Input: part model. Units: mm. Frame: model coordinates. A direction names the side the tool comes from. Round coordinates to 2 decimals unless told otherwise and drop trailing zeros. Loops run counter-clockwise (first coordinate to the right, second up) from the corner with the lowest first, then second, coordinate; pieces in that order, holes last.
1) Access query for faces 5 (the face through (13.756, -19.825, 6.261)), 6 (the face through (-20, -6.35, 6)). Directions: +Z, -Z, +X, -X, +Y, -Y. A direction counts if a zero-diameter tool reaches every point of the face in a straight line with its end or side. Return the directions, or none.
2) Section C-C, the plane z = 6.75. Return loops of the section in (x, y), and give its area (3 significant figures).
3) Section B-B, the plane y = -11. Return loops of the section in (x, z).
4) Section D-D, the plane y = 0. Return loops of the section in (x, z), and give its area (3 significant figures).
5) Ray query, line 1 along Y through (x, z) = (0, 4); line 2 along Y through (x, z) = (-18.5, 4.5); line 3 along X through (y, z) = (0, 8). Return the intervals inside material, ascending.
6) Section A-A, the plane x = 0. Return loops of the section in (y, z), and give its area (3 significant figures).
7) First-contact query: pin 1 (7.5 mm diameter, centred on x = -19.5, z = 9, fed in from -Y); pin 2 (1.5 mm diameter, centred on x = 9, z = 1.5, fed in from -Y); pin 3 (2 mm diameter, centred on x = -18.5, z = 8.5, fed in from +Y); pin 4 (6 mm diameter, centred on x = -15, y = -17, fed in from -Z). Flat tips, straight axial feed; report the tip coordinate or a pass-through.
8) Draft query along Y for faces 1 (the face through (-20, 6.35, 6)), 2 (the face through (0, 20.32, 6)), 3 (the face through (16, -8, 12.7)), 4 (the face through (17.487, 0.679, 6.261)). Return one class per face: pulls with the +Y half, pulls with the -Y half, needs draft (parallel to the pull), parting line crosses it, or undercut.
from build123d import *

# Parameters (mm, degrees)
F1_DEPTH = 12.7


with BuildPart() as f1:
    # F0 (on Top) → F1 (new body)
    with BuildSketch(Plane.XY):
        with BuildLine():
            ThreePointArc((-16.307928, 6.35), (17.5006, 0), (-16.307928, -6.35))
            Line((-16.307928, -6.35), (-23.279485, -6.35))
            ThreePointArc((-23.279485, -6.35), (14.288778, -19.444478), (13.013627, 20.32))
            Line((13.013627, 20.32), (-13.013627, 20.32))
            ThreePointArc((-13.013627, 20.32), (-19.444478, 14.288778), (-23.279485, 6.35))
            Line((-23.279485, 6.35), (-16.307928, 6.35))
        make_face()
    extrude(amount=F1_DEPTH)


solid = f1.part
Final values:
1. face 5: +Z, -Z
1. face 6: +Z, -Z, -X
2. outline: (-23.28, -6.35) arc R24.13 ccw (long way) to (13.01, 20.32) - (-13.01, 20.32) arc R24.13 ccw to (-23.28, 6.35) - (-16.31, 6.35) arc R17.5 cw (long way) to (-16.31, -6.35) - close
2. area: 714 mm2
3. outline: (-21.48, 0) - (-13.61, 0) - (-13.61, 12.7) - (-21.48, 12.7) - close; (13.61, 0) - (21.48, 0) - (21.48, 12.7) - (13.61, 12.7) - close
4. outline: (17.5, 0) - (24.13, 0) - (24.13, 12.7) - (17.5, 12.7) - close
4. area: 84.2 mm2
5. line 1: y = -24.13 to -17.5, 17.5 to 20.32
5. line 2: y = -15.49 to -6.35, 6.35 to 15.49
5. line 3: x = 17.5 to 24.13
6. outline: (-24.13, 0) - (-17.5, 0) - (-17.5, 12.7) - (-24.13, 12.7) - close; (17.5, 0) - (20.32, 0) - (20.32, 12.7) - (17.5, 12.7) - close
6. area: 120 mm2
7. pin 1: stops at y = -18.28
7. pin 2: stops at y = -22.68
7. pin 3: stops at y = 16.61
7. pin 4: stops at z = 0
8. face 1: undercut
8. face 2: pulls with the +Y half
8. face 3: needs draft
8. face 4: undercut
